Part model, mm, in its own coordinate system. Round coordinates to 2 decimals unless told otherwise and drop trailing zeros. Write each loop counter-clockwise with the first axis right and the second up, starting at its lowest first coordinate (ties: lowest second). Pieces come first, ordered by that corner, then holes.
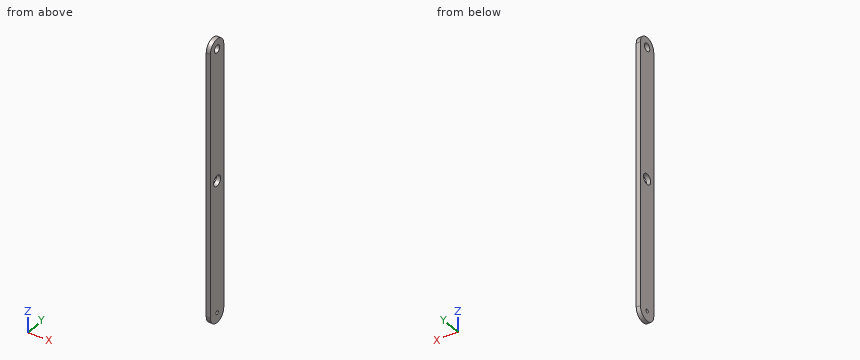
from build123d import *

# Parameters (mm, degrees)
SKETCH1_R             = 3
SKETCH1_R_2           = 4
BOSS_EXTRUDE1_DEPTH   = 3.175
F_6_32_TAPPED_HOLE1_D = 2.7051


with BuildPart() as part:
    # Sketch1 → Boss-Extrude1 (new body)
    with BuildSketch(Plane(origin=(0, 0, 0), x_dir=(0, 0, -1), z_dir=(1, 0, 0))):
        with BuildLine():
            Line((-100, 7.5), (100, 7.5))
            ThreePointArc((100, 7.5), (107.5, 0), (100, -7.5))
            Line((100, -7.5), (-100, -7.5))
            ThreePointArc((-100, -7.5), (-107.5, 0), (-100, 7.5))
        make_face()
        with Locations((-100, 0)):
            Circle(SKETCH1_R, mode=Mode.SUBTRACT)
        Circle(SKETCH1_R_2, mode=Mode.SUBTRACT)
    extrude(amount=BOSS_EXTRUDE1_DEPTH)

    # #6-32 Tapped Hole1 (through all)
    with Locations(Plane(origin=(3.175, 0, 0), x_dir=(0, 0, -1), z_dir=(1, 0, 0))):
        with Locations((100, 0)):
            Hole(F_6_32_TAPPED_HOLE1_D / 2)


solid = part.part
Q1. Saw through at C-C, the plane y = 5.75. Write the cut outline in (x, z) (3 decimals).
Q2. Wall check: line 1 (Y direction, x = 1.9, z = 100); line 2 (Y direction, x = 2.55, z = -100); line 3 (Z direction, x = 1.9, y = -2). Give the ranges that are in metal, low to high.
Q3. Saw through at B-B, the plane z = 0. Write the cut outline in (x, y) (3 decimals), and give its area (3 significant figures).
Q4. Drop flat-ended pins along their axis: P1, Ø7, axis at y = 0, z = 0, coming from the -X side; P2, Ø1, axis at x = 1, y = -5, coming from the +Z side. Give the stop position or say it passes through.
Q5. Saw through at A-A, the plane x = 1.45. Write the cut outline in (y, z).
Computed:
1. outline: (0, -104.815) - (3.175, -104.815) - (3.175, 104.815) - (0, 104.815) - close
2. line 1: y = -7.5 to -3, 3 to 7.5
2. line 2: y = -7.5 to -1.35, 1.35 to 7.5
2. line 3: z = -107.23 to -3.46, 3.46 to 97.76, 102.24 to 107.23
3. outline: (0, -7.5) - (3.175, -7.5) - (3.175, -4) - (0, -4) - close; (0, 4) - (3.175, 4) - (3.175, 7.5) - (0, 7.5) - close
3. area: 22.2 mm2
4. P1: passes through
4. P2: stops at z = 106
5. outline: (-7.5, -100) arc R7.5 ccw to (7.5, -100) - (7.5, 100) arc R7.5 ccw to (-7.5, 100) - close; hole circle Ø8 at (0, 0); hole circle Ø6 at (0, 100); hole circle Ø2.71 at (0, -100)
